The listing builds one solid part. Answer for the finished solid, in the listing's coordinates (mm). A direction names the side the tool comes from. Give positions to 0.01 mm unless a question says otherwise; leave off trailing zeros. Order: outer loops, then holes, each group sorted by start corner. A loop starts at its lowest first (then second) coordinate and runs counter-clockwise, first axis right, second up. Notation, with made-up numbers: M 53,26 L 72,26 A32 ccw 72,62 Z; hole C 29,25.25 d8. An arc over 180 degrees is marked long. Answer as a JSON object with one key per item and string values. Group by question number.
Autodesk Fusion 360 part; units mm, degrees
sketch "Sketch1" plane through (0, 0, 0) normal (0, 1, 0) x (1, 0, 0)
  line L0 (0, 0) -> (23, 0)
  line L1 (23, 0) -> (23, -150)
  line L2 (23, -150) -> (0, -150)
  line L3 (0, -150) -> (0, 0)
  dimension "d1" = 23
  dimension "d2" = 150
extrude "Extrude1" add sketch "Sketch1" along normal blind 6.43
sketch "Sketch2" plane through (0, 6.43, 0) normal (0, 1, 0) x (1, 0, 0)
  line L0 (11.5, 0) -> (11.5, -150) construction
  line L1 (0, 0) -> (0, -150)
  line L2 (0, -75) -> (23, -75) construction
  line L3 (19, -70) -> (4, -70) construction
  line L4 (4, -70) -> (4, -80) construction
  line L5 (4, -80) -> (19, -80) construction
  line L6 (19, -80) -> (19, -70) construction
  line L7 (19, -70) -> (4, -80) construction
  line L8 (4, -70) -> (19, -80) construction
  line L9 (23, 0) -> (0, 0)
  line L10 (0, -150) -> (23, -150)
  line L11 (0, -150) -> (23, -150)
  line L12 (23, -150) -> (23, 0)
  line L13 (23, 0) -> (0, 0)
  line L14 (0, 0) -> (0, -150)
  point P0 (11.5, -75)
  point P1 (4, -70)
  point P2 (19, -70)
  point P3 (19, -80)
  point P4 (4, -80)
  point P5 (3.7, -7.25)
  point P6 (19.3, -7.25)
  point P7 (3.7, -33.92)
  point P8 (3.7, -60.59)
  point P9 (3.7, -87.26)
  point P10 (19.3, -33.92)
  point P11 (19.3, -60.59)
  point P12 (19.3, -87.26)
  dimension "d5" = 11.5
  dimension "d6" = 15
  dimension "d7" = 10
  dimension "d8" = 15.6
  dimension "d9" = 19.3
  dimension "d10" = 7.25
  dimension "d13" = 0
  dimension "d14" = -26.67
  dimension "d17" = 0
  dimension "d18" = -26.67
hole "Hole1" at (4, 6.43, 70) direction (0, -1, 0) diameter 3.4 end through all counterbore diameter 6.5 counterbore depth 3
hole "Hole2" at (19, 6.43, 70) direction (0, -1, 0) diameter 3.4 end through all counterbore diameter 6.5 counterbore depth 3
hole "Hole3" at (4, 6.43, 80) direction (0, -1, 0) diameter 3.4 end through all counterbore diameter 6.5 counterbore depth 3
hole "Hole4" at (19, 6.43, 80) direction (0, -1, 0) diameter 3.4 end through all counterbore diameter 6.5 counterbore depth 3
hole "Hole5" at (3.7, 6.43, 7.25) direction (0, -1, 0) diameter 2.05 end through all
hole "Hole6" at (19.3, 6.43, 7.25) direction (0, -1, 0) diameter 2.05 end through all
hole "Hole7" at (3.7, 6.43, 33.92) direction (0, -1, 0) diameter 2.05 end through all
hole "Hole8" at (19.3, 6.43, 33.92) direction (0, -1, 0) diameter 2.05 end through all
hole "Hole9" at (3.7, 6.43, 60.59) direction (0, -1, 0) diameter 2.05 end through all
hole "Hole10" at (19.3, 6.43, 60.59) direction (0, -1, 0) diameter 2.05 end through all
hole "Hole11" at (3.7, 6.43, 87.26) direction (0, -1, 0) diameter 2.05 end through all
hole "Hole12" at (19.3, 6.43, 87.26) direction (0, -1, 0) diameter 2.05 end through all
sketch "Sketch3" plane through (0, 0, 0) normal (0, -1, 0) x (1, 0, 0)
  circle A0 centre (19.3, 87.26) radius 1.025
  circle A1 centre (3.7, 87.26) radius 1.025
  circle A2 centre (19.3, 60.59) radius 1.025
  circle A3 centre (3.7, 60.59) radius 1.025
  circle A4 centre (19.3, 33.92) radius 1.025
  circle A5 centre (3.7, 33.92) radius 1.025
  circle A6 centre (19.3, 7.25) radius 1.025
  circle A7 centre (3.7, 7.25) radius 1.025
  circle A8 centre (19, 80) radius 1.7
  circle A9 centre (4, 80) radius 1.7
  circle A10 centre (19, 70) radius 1.7
  circle A11 centre (4, 70) radius 1.7
  line L0 (23, 150) -> (0, 150)
  line L1 (0, 150) -> (0, 0)
  line L2 (0, 0) -> (23, 0)
  line L3 (23, 0) -> (23, 150)
  line L4 (0, 150) -> (23, 150)
  point P0 (15.6, 140)
  point P1 (7.46, 140)
  dimension "d92" = 8.14
  dimension "d93" = 10
  dimension "d94" = 7.4
hole "Hole17" at (7.4, 0, 140) direction (0, 1, 0) diameter 3.4 end through all counterbore diameter 6.5 counterbore depth 3
hole "Hole18" at (15.54, 0, 140) direction (0, 1, 0) diameter 3.4 end through all counterbore diameter 6.5 counterbore depth 3
Item 1: Section B-B (z = 70) is taken. Determine the outline of the cut face in (x, y), and give its area (3 significant figures).
Item 2: A tool of negligible diameter and unlimited length cuts with its end or side. For faces 1 (the flat face through (9, 3, 139)), 2 (the flat face through (5.4, 3.43, 81.4)), 3 (the flat face through (11, 0, 74)), from which of +Z, -Z, +X, -X, +Y, -Y can it reach the whole face along a straight path? Write none if from no direction.
Item 3: Section A-A (y = 4.5) is taken. Count the separate pieces of the cut face and the enclosed holes in it, and give its area (3 significant figures).
Item 4: Consider probe 1 along X at (y, z) = (4.4, 70); probe 2 along X at (y, z) = (1.75, 33.92) (3 decimals); probe 3 along Z at (x, y) = (2.25, 4.5). Determine where each line is inside the solid, lowest interval first. Write a range as from..to.
Item 5: A flat-ended cylindrical pin translates along its axis: P1, Ø4.5, axis at x = 4, z = 80, coming from the +Y side. Find the tip coordinate at first contact, or state that the pin passes through.
Item 6: Determine the mould class of faces 4 (the cylindrical face through (15.03, 4.74, 138.38)), 5 (the flat face through (12, 3, 150)) for opening direction X: released by +X, released by -X, zero draft, split by the parting line, or undercut.
Values found:
{
 "1": {"outline": "M 0,0 L 2.3,0 L 2.3,3.43 L 0.75,3.43 L 0.75,6.43 L 0,6.43 Z; M 5.7,0 L 17.3,0 L 17.3,3.43 L 15.75,3.43 L 15.75,6.43 L 7.25,6.43 L 7.25,3.43 L 5.7,3.43 Z; M 20.7,0 L 23,0 L 23,6.43 L 22.25,6.43 L 22.25,3.43 L 20.7,3.43 Z", "area": "85.6 mm^2"},
 "2": {"face 1": "-Y", "face 2": "+Y", "face 3": "+Z, -Z, +X, -X, -Y"},
 "3": {"separate pieces": "1", "enclosed holes": "14", "area": "3,270 mm^2"},
 "4": {"probe 1": "x = 0..0.75, 7.25..15.75, 22.25..23", "probe 2": "x = 0..2.675, 4.725..18.275, 20.325..23", "probe 3": "z = 0..67.26, 72.74..77.26, 82.74..150"},
 "5": {"P1": "stops at y = 3.43"},
 "6": {"face 4": "undercut", "face 5": "zero draft"}
}
